from build123d import *

# Parameters (mm, degrees)
SKETCH1_W                                           = 25.41
SKETCH1_H                                           = 18.5
BOSS_EXTRUDE1_DEPTH                                 = 12
F_2_56_TAPPED_HOLE1_D                               = 1.778
F_2_56_TAPPED_HOLE1_DEPTH                           = 7.46583491
F_2_56_TAPPED_HOLE1_TIP                             = 0.53416509
SKETCH5_R                                           = 3
CUT_EXTRUDE1_DEPTH                                  = 3
CBORE_FOR_2_BINDING_HEAD_MACHINE_SCREW3_D           = 2.4384
CBORE_FOR_2_BINDING_HEAD_MACHINE_SCREW3_CBORE_D     = 5.55752
CBORE_FOR_2_BINDING_HEAD_MACHINE_SCREW3_CBORE_DEPTH = 7.269988


with BuildPart() as part:
    # Sketch1 → Boss-Extrude1 (new body)
    with BuildSketch(Plane(origin=(0, 0, 0), x_dir=(1, 0, 0), z_dir=(0, 1, 0))):
        with Locations((12.705, 9.25)):
            Rectangle(SKETCH1_W, SKETCH1_H)
    extrude(amount=BOSS_EXTRUDE1_DEPTH)

    # #2-56 Tapped Hole1
    with Locations(Plane(origin=(0, 0, 0), x_dir=(-1, 0, 0), z_dir=(0, -1, 0))):
        with Locations((-23.91, 17), (-23.91, 1.5), (-1.5, 1.5), (-1.5, 17)):
            Hole(F_2_56_TAPPED_HOLE1_D / 2, depth=F_2_56_TAPPED_HOLE1_DEPTH)
            with Locations((0, 0, -(F_2_56_TAPPED_HOLE1_DEPTH + F_2_56_TAPPED_HOLE1_TIP / 2))):  # 118° drill point
                Cone(0, F_2_56_TAPPED_HOLE1_D / 2, F_2_56_TAPPED_HOLE1_TIP, mode=Mode.SUBTRACT)

    # Sketch5 → Cut-Extrude1 (cut)
    with BuildSketch(Plane.XZ):
        with Locations((12.705, -9.25)):
            Circle(SKETCH5_R)
    extrude(amount=-CUT_EXTRUDE1_DEPTH, mode=Mode.SUBTRACT)

    # CBORE for #2 Binding Head Machine Screw3 (through all)
    with Locations(Plane(origin=(0, 0, 0), x_dir=(-1, 0, 0), z_dir=(0, -1, 0))):
        with Locations((-12.705, 17), (-12.705, 1.5)):
            CounterBoreHole(CBORE_FOR_2_BINDING_HEAD_MACHINE_SCREW3_D / 2, CBORE_FOR_2_BINDING_HEAD_MACHINE_SCREW3_CBORE_D / 2, CBORE_FOR_2_BINDING_HEAD_MACHINE_SCREW3_CBORE_DEPTH)


solid = part.part
The model under review builds one solid part; all positions refer to its coordinate system, in mm. A direction names the side the tool comes from. Round coordinates to 2 decimals unless told otherwise and drop trailing zeros. Write each loop counter-clockwise with the first axis right and the second up, starting at its lowest first coordinate (ties: lowest second). Pieces come first, ordered by that corner, then holes. Notation, with made-up numbers: M 55.5,-3.75 L 69.5,-3.75 A20 ccw 69.5,27.25 Z; hole C -23.5,47 d10. An arc over 180 degrees is marked long. Use a Markdown table: item, result. Add a question column.
Q1. We need section D-D, the plane y = 2.25. State the section outline as (x, z) points (3 decimals).
Q2. We need section B-B, the plane y = 11.25. State the section outline as (x, z) points (3 decimals).
Q3. Insertion check: pin 1 (3.5 mm diameter, centred on x = 13, z = -16.5, fed in from -Y); pin 2 (3.5 mm diameter, centred on x = 12.705, z = -9.25, fed in from -Y). Each pin has a flat end and moves straight along its axis. Give the tip position at first contact, or say it passes through.
Q4. We need section A-A, the plane z = -9.25. State the section outline as (x, y) points (3 decimals), plus the area to 3 significant figures.
Q5. We need section C-C, the plane y = 6. State the section outline as (x, z) points (3 decimals).
Q6. Machinability: for faces 1 (the face through (0, 6, -9)), 2 (the face through (12, 7.27, -3)), which of the approach directions +Z, -Z, +X, -X, +Y, -Y give a long, thin tool a straight path to every point of the face, cutting with its end or side? Answer none if there is none.
Q7. To check wall thickness, follow line 1 (X direction, y = 4.75, z = -17); line 2 (Z direction, x = 1.25, y = 5.5); line 3 (X direction, y = 10.05, z = -17). State the ranges of each line that lie inside material, in increasing order.
Findings below:
| question | item | result |
|---|---|---|
| 1 | outline | M 0,-18.5 L 10.366,-18.5 A2.779 cw long 15.044,-18.5 L 25.41,-18.5 L 25.41,0 L 15.044,0 A2.779 cw long 10.366,0 L 0,0 Z; hole C 1.5,-17 d1.778; hole C 1.5,-1.5 d1.778; hole C 12.705,-9.25 d6; hole C 23.91,-17 d1.778; hole C 23.91,-1.5 d1.778 |
| 2 | outline | M 0,-18.5 L 25.41,-18.5 L 25.41,0 L 0,0 Z; hole C 12.705,-17 d2.438; hole C 12.705,-1.5 d2.438 |
| 3 | pin 1 | stops at y = 7.27 |
| 3 | pin 2 | stops at y = 3 |
| 4 | outline | M 0,0 L 9.705,0 L 9.705,3 L 15.705,3 L 15.705,0 L 25.41,0 L 25.41,12 L 0,12 Z |
| 4 | area | 287 mm² |
| 5 | outline | M 0,-18.5 L 10.366,-18.5 A2.779 cw long 15.044,-18.5 L 25.41,-18.5 L 25.41,0 L 15.044,0 A2.779 cw long 10.366,0 L 0,0 Z; hole C 1.5,-17 d1.778; hole C 1.5,-1.5 d1.778; hole C 23.91,-17 d1.778; hole C 23.91,-1.5 d1.778 |
| 6 | face 1 | +Z, -Z, -X, +Y, -Y |
| 6 | face 2 | -Y |
| 7 | line 1 | x = 0 to 0.61, 2.39 to 9.93, 15.48 to 23.02, 24.8 to 25.41 |
| 7 | line 2 | z = -18.5 to -17.85, -16.15 to -2.35, -0.65 to 0 |
| 7 | line 3 | x = 0 to 11.49, 13.92 to 25.41 |
